For this review, use the dimensioned drawing (mm, ordinates from the lowest corner) and the shaded views. A direction names the side the tool comes from. Round coordinates to 2 decimals unless told otherwise and drop trailing zeros. Loops run counter-clockwise (first coordinate to the right, second up) from the corner with the lowest first, then second, coordinate; pieces in that order, holes last. Notation, with made-up numbers: M -6.5,6 L 47.5,6 A20 cw 47.5,36 Z; hole C -21.5,11 d7. An arc over 180 degrees is marked long. Write item = value, one per line. Start each with the question number.
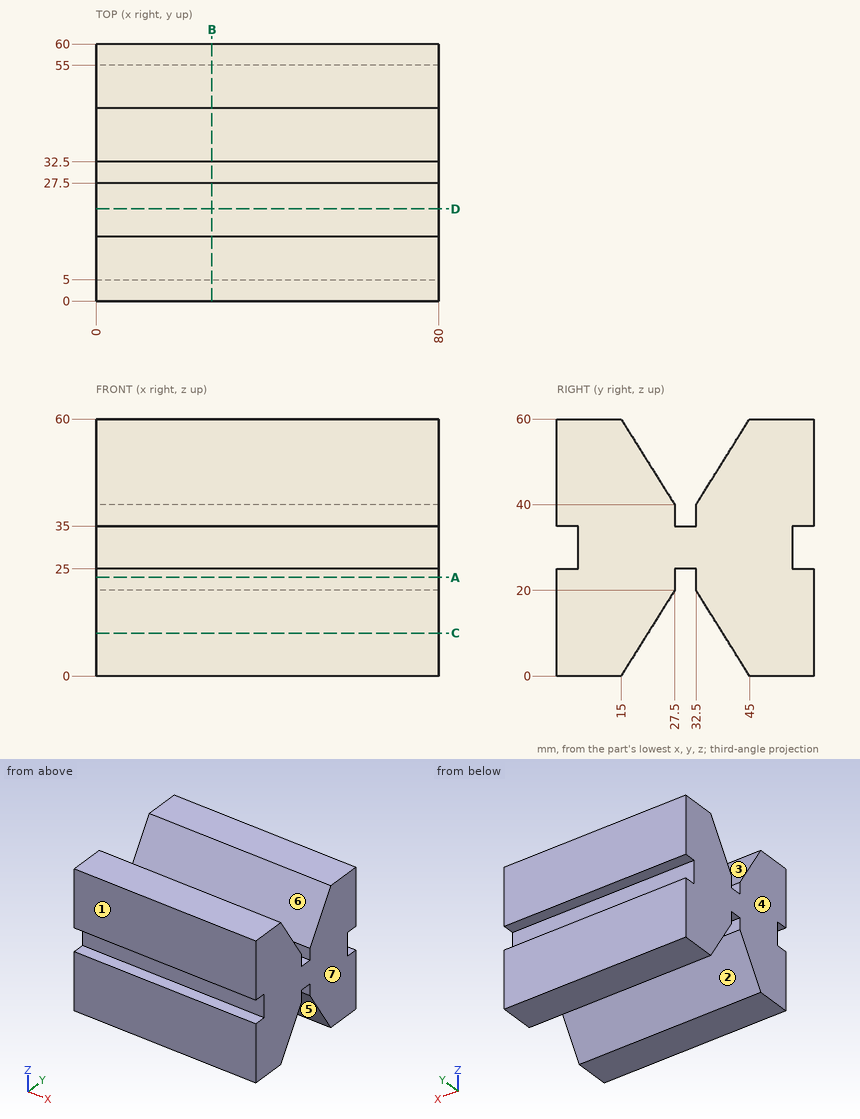
(1) Add section B-B on x = 27. Write out the cut boundary in (y, z).
(2) Add section A-A on z = 23. Write out the cut boundary in (x, y), and give its area (3 significant figures).
(3) Wall thickness on L1, parallel to Y at x = 70.5, z = 38; L2, parallel to Y at x = 75.5, z = 52; L3, parallel to Y at x = 30, z = 26: over which ranges is each line inside the solid? List them lowest first.
(4) Add section D-D on y = 21.5. Write out the cut boundary in (x, z).
(5) Draft analysis for pull direction Y (two halves, no side actions). For the marked faces 1, 2, 3 and 4, state which applies: +Y half, -Y half, draft (parallel to the pull), parting line (faces both ways), or undercut.
(6) Tool access review of the marked faces 5, 6 and 7: name each direction out of +Z, -Z, +X, -X, +Y, -Y from which nothing blocks a thin tool from reaching the whole face with its end or side.
(7) For pin 1 Ø5 at (x, z) = (37, 29.5) entering from +Y; pin 2 Ø3 at (x, y) = (32.5, 16) entering from -Z; pin 3 Ø4 at (x, y) = (56.5, 30) entering from -Z; pin 4 Ø1.5 at (x, y) = (57, 31) entering from +Z, all flat-tipped, find the tip position at first contact; note any pin that passes through.
(8) Add section C-C on z = 10. Write out the cut boundary in (x, y), and give its area (3 significant figures).
Answer sheet:
q1.outline = M 0,0 L 15,0 L 27.5,20 L 27.5,25 L 32.5,25 L 32.5,20 L 45,0 L 60,0 L 60,25 L 55,25 L 55,35 L 60,35 L 60,60 L 45,60 L 32.5,40 L 32.5,35 L 27.5,35 L 27.5,40 L 15,60 L 0,60 L 0,35 L 5,35 L 5,25 L 0,25 Z
q2.outline = M 0,0 L 80,0 L 80,27.5 L 0,27.5 Z; M 0,32.5 L 80,32.5 L 80,60 L 0,60 Z
q2.area = 4,400 mm²
q3.L1 = 0 to 27.5, 32.5 to 60
q3.L2 = 0 to 20, 40 to 60
q3.L3 = 5 to 55
q4.outline = M 0,10.4 L 80,10.4 L 80,49.6 L 0,49.6 Z
q5.face_1 = -Y half
q5.face_2 = undercut
q5.face_3 = undercut
q5.face_4 = draft
q6.face_5 = -Z, +X, -X
q6.face_6 = +Z, +X, -X
q6.face_7 = +Z, -Z, +X, +Y, -Y
q7.pin_1 = 55
q7.pin_2 = 0
q7.pin_3 = 25
q7.pin_4 = 35
q8.outline = M 0,0 L 80,0 L 80,21.25 L 0,21.25 Z; M 0,38.75 L 80,38.75 L 80,60 L 0,60 Z
q8.area = 3,400 mm²
